The listing builds one solid part. Answer for the finished solid, in the listing's coordinates (mm). A direction names the side the tool comes from. Round coordinates to 2 decimals unless told otherwise and drop trailing zeros. Loops run counter-clockwise (first coordinate to the right, second up) from the corner with the lowest first, then second, coordinate; pieces in that order, holes last. Notation, with made-up numbers: (87, 37.5) -> (116, 37.5) arc R17 cw to (116, 63.5) -> close; hole circle Ø5 at (29.25, 43). An arc over 180 degrees is marked (long way). One line per question, with ' | ' between items.
from build123d import *

# Parameters (mm, degrees)
BOSS_EXTRUDE1_DEPTH = 5
SKETCH2_R           = 1.608
CUT_EXTRUDE1_DEPTH  = 58.548241502
FILLET1_R           = 0.994


with BuildPart() as part:
    # Sketch1 → Boss-Extrude1 (new body)
    with BuildSketch(Plane(origin=(0, 0, 0), x_dir=(1, 0, 0), z_dir=(0, 1, 0))):
        Polygon((-50.76, -26.65), (-50.76, 26.65), (44.689, 26.65), (47.228, 24.111), (47.228, 13.955), (50.76, 10.423), (50.76, -23.834), (48.221, -26.373), (48.221, -26.65), align=None)
    extrude(amount=BOSS_EXTRUDE1_DEPTH)

    # Sketch2 → Cut-Extrude1 (cut, through all)
    with BuildSketch(Plane(origin=(0, 0, 0), x_dir=(1, 0, 0), z_dir=(0, 1, 0))):
        with Locations(Location((-35.525, 24.111, 0), (0, 0, 270))):
            Circle(SKETCH2_R)
        with Locations(Location((-36.795, -24.111, 0), (0, 0, 270))):
            Circle(SKETCH2_R)
        with Locations(Location((15.235, 8.876, 0), (0, 0, 270))):
            Circle(SKETCH2_R)
        with Locations(Location((15.235, -19.033, 0), (0, 0, 270))):
            Circle(SKETCH2_R)
        with Locations(Location((39.357, 24.111, 0), (0, 0, 270))):
            Circle(SKETCH2_R)
        with Locations(Location((45.684, -24.111, 0), (0, 0, 270))):
            Circle(SKETCH2_R)
    extrude(amount=CUT_EXTRUDE1_DEPTH, mode=Mode.SUBTRACT)

    # Fillet1
    # the kernel refuses this fillet: 0.994 mm, written as the material it takes off along each edge
    with BuildSketch(Plane(origin=(48.221, -1.721095218, 26.65), x_dir=(-1, 0, 0), z_dir=(0, 1, 0))) as fillet1_piece_1:
        with BuildLine():
            CenterArc((0.688438087, -0.994), FILLET1_R, 90, 43.83577097)
            Line((0, -0.277), (-0.013768762, -0.26266))
            ThreePointArc((-0.013768762, -0.26266), (-0.01988, -0.1385), (-0.01988, 0))
            Line((-0.01988, 0), (0, 0.01988))
            Line((0, 0.01988), (0.688438087, 0.01988))
            Line((0.688438087, 0.01988), (0.688438087, 0))
        make_face()
    extrude(amount=8.442190436, mode=Mode.SUBTRACT)
    with BuildSketch(Plane(origin=(-50.76, -2.485, 26.65), x_dir=(0, 0, -1), z_dir=(0, 1, 0))) as fillet1_piece_2:
        with BuildLine():
            CenterArc((FILLET1_R, -FILLET1_R), FILLET1_R, 90, 90)
            Line((0, -FILLET1_R), (-FILLET1_R * 0.02, -FILLET1_R))
            Line((-FILLET1_R * 0.02, -FILLET1_R), (-FILLET1_R * 0.02, FILLET1_R * 0.02))
            Line((-FILLET1_R * 0.02, FILLET1_R * 0.02), (FILLET1_R, FILLET1_R * 0.02))
            Line((FILLET1_R, FILLET1_R * 0.02), (FILLET1_R, 0))
        make_face()
    extrude(amount=9.97, mode=Mode.SUBTRACT)
    with BuildSketch(Plane(origin=(-50.76, -2.485, -26.65), x_dir=(0, 0, 1), z_dir=(0, 1, 0))) as fillet1_piece_3:
        with BuildLine():
            CenterArc((FILLET1_R, FILLET1_R), FILLET1_R, 180, 90)
            Line((0, FILLET1_R), (-FILLET1_R * 0.02, FILLET1_R))
            Line((-FILLET1_R * 0.02, FILLET1_R), (-FILLET1_R * 0.02, -FILLET1_R * 0.02))
            Line((-FILLET1_R * 0.02, -FILLET1_R * 0.02), (FILLET1_R, -FILLET1_R * 0.02))
            Line((FILLET1_R, -FILLET1_R * 0.02), (FILLET1_R, 0))
        make_face()
    extrude(amount=9.97, mode=Mode.SUBTRACT)


solid = part.part
Q1. Given pin 1 Ø3 at (x, z) = (-35.525, -24.111) entering from -Y, flat-ended and moving along its own axis, determine where the tip first touches the part or whether it passes through.
Numbers:
pin 1: through
Q2. A cutting plane is placed at A-A on y = 0.95. Give the vertices of the cut face in (x, z) (3 decimals).
Numbers:
outline: (-50.76, -25.656) arc R0.994 ccw to (-49.766, -26.65) -> (44.689, -26.65) -> (47.228, -24.111) -> (47.228, -13.955) -> (50.76, -10.423) -> (50.76, 23.834) -> (48.221, 26.373) arc R0.994 ccw to (47.533, 26.65) -> (-49.766, 26.65) arc R0.994 ccw to (-50.76, 25.656) -> close; hole circle Ø3.216 at (-36.795, 24.111); hole circle Ø3.216 at (-35.525, -24.111); hole circle Ø3.216 at (15.235, -8.876); hole circle Ø3.216 at (15.235, 19.033); hole circle Ø3.216 at (39.357, -24.111); hole circle Ø3.216 at (45.684, 24.111)
Q3. Find the intervals of material crossed by line 1 (X direction, y = 0.6, z = -9); line 2 (X direction, y = 1, z = -17); line 3 (Z direction, x = -38, y = 4.35), in increasing order. Write a range as from..to.
Numbers:
line 1: -50.76..13.63, 16.84..50.76 | line 2: -50.76..47.23 | line 3: -26.65..23.05, 25.18..26.65
Q4. A cutting plane is placed at B-B on z = -21.5. Give the vertices of the cut face in (x, y).
Numbers:
outline: (-50.76, 0) -> (47.23, 0) -> (47.23, 5) -> (-50.76, 5) -> close
Q5. For faces 1 (the face through (44.257, 2.465, 24.853)), 2 (the face through (47.228, 2, -19)), determine the directions among +Z, -Z, +X, -X, +Y, -Y from which every point of the face is accessible in a straight line to the end or side of a thin tool.
Numbers:
face 1: +Y, -Y | face 2: -Z, +X, +Y, -Y
Q6. A cutting plane is placed at C-C on z = -12. Give the vertices of the cut face in (x, y), plus the area to 3 significant figures.
Numbers:
outline: (-50.76, 0) -> (49.18, 0) -> (49.18, 5) -> (-50.76, 5) -> close | area: 500 mm^2
Q7. For a pull along Z with two mould halves and no side action, classify faces 3 (the face through (-38.222, 2.465, 24.853)), 4 (the face through (48.969, 2.465, -12.214)), 5 (the face through (1, 0, 0)) as pulls with the +Z half, pulls with the -Z half, needs draft (parallel to the pull), parting line crosses it, or undercut.
Numbers:
face 3: undercut | face 4: pulls with the -Z half | face 5: needs draft
